For this review, take the finished solid that the model builds, in its own axes (mm). A direction names the side the tool comes from. Give positions to 0.01 mm unless a question says otherwise; leave off trailing zeros. Loops run counter-clockwise (first coordinate to the right, second up) from the corner with the lowest first, then second, coordinate; pieces in that order, holes last.
```python
from build123d import *

# Parameters (mm, degrees)
SKETCH2_W           = 45
SKETCH2_H           = 45
SKETCH2_R           = 11.5
SKETCH2_R_2         = 7.5
BOSS_EXTRUDE1_DEPTH = 4
SKETCH2_3_R         = 11.5
SKETCH2_3_R_2       = 7.5
BOSS_EXTRUDE2_DEPTH = 46
CHAMFER1_SIZE       = 10
SKETCH3_W           = 7
SKETCH3_H           = 20.450898806
CUT_EXTRUDE1_DEPTH  = 19


with BuildPart() as part:
    # Sketch2 → Boss-Extrude1 (new body)
    # profile 1 of 3: a face of its own
    with BuildSketch(Plane(origin=(0, 0, 0), x_dir=(1, 0, 0), z_dir=(0, 1, 0))):
        Rectangle(SKETCH2_W, SKETCH2_H)
        Circle(SKETCH2_R, mode=Mode.SUBTRACT)
    # profile 2 of 3: a face of its own
    with BuildSketch(Plane(origin=(0, 0, 0), x_dir=(1, 0, 0), z_dir=(0, 1, 0))):
        Circle(SKETCH2_R)
        Circle(SKETCH2_R_2, mode=Mode.SUBTRACT)
    # profile 3 of 3: a face of its own
    with BuildSketch(Plane(origin=(0, 0, 0), x_dir=(1, 0, 0), z_dir=(0, 1, 0))):
        Circle(SKETCH2_R_2)
    extrude(amount=-BOSS_EXTRUDE1_DEPTH)

    # Sketch2_3 → Boss-Extrude2 (add)
    with BuildSketch(Plane(origin=(0, 0, 0), x_dir=(1, 0, 0), z_dir=(0, 1, 0))):
        with Locations(Location((0, 0, 0), (0, 0, 270))):
            Circle(SKETCH2_3_R)
        with Locations(Location((0, 0, 0), (0, 0, 270))):
            Circle(SKETCH2_3_R_2, mode=Mode.SUBTRACT)
    extrude(amount=BOSS_EXTRUDE2_DEPTH)

    # Chamfer1
    chamfer1_edges = [part.edges().sort_by_distance(p)[0] for p in [
        (0, 0, -11.5),
    ]]
    chamfer(chamfer1_edges, length=CHAMFER1_SIZE)

    # Sketch3 → Cut-Extrude1 (cut)
    with BuildSketch(Plane.XY):
        with Locations((0, 21.362604589)):
            Rectangle(SKETCH3_W, SKETCH3_H)
    extrude(amount=CUT_EXTRUDE1_DEPTH, mode=Mode.SUBTRACT)


solid = part.part
```
Q1. Consider section A-A on x = 0. Give the boundary of the cut face in (y, z).
Answers:
outline: (-4, -22.5) - (0, -22.5) - (0, -21.5) - (10, -11.5) - (46, -11.5) - (46, -7.5) - (0, -7.5) - (0, 7.5) - (11.14, 7.5) - (11.14, 11.5) - (10, 11.5) - (0, 21.5) - (0, 22.5) - (-4, 22.5) - close; (31.59, 7.5) - (46, 7.5) - (46, 11.5) - (31.59, 11.5) - close
Q2. Consider section B-B on z = 0. Give the boundary of the cut face in (x, y).
Answers:
outline: (-22.5, -4) - (22.5, -4) - (22.5, 0) - (21.5, 0) - (11.5, 10) - (11.5, 46) - (7.5, 46) - (7.5, 0) - (-7.5, 0) - (-7.5, 46) - (-11.5, 46) - (-11.5, 10) - (-21.5, 0) - (-22.5, 0) - close
Q3. For probe 1 along X at (y, z) = (11, 0); probe 2 along Y at (x, z) = (19.5, 20); probe 3 along X at (y, z) = (17, 4), list the stretches that pass through material, from the lowest coordinate up.
Answers:
probe 1: x = -11.5 to -7.5, 7.5 to 11.5
probe 2: y = -4 to 0
probe 3: x = -10.78 to -6.34, 6.34 to 10.78
Q4. Mouldability with a two-part tool opening along Y and no side actions: class faces 4 (the flat face through (0, 11.137, 9)), 5 (the flat face through (0, 0, 0)), 6 (the flat face through (0, -4, 0)) as +Y half, -Y half, draft (parallel to the pull), parting line (faces both ways), or undercut.
Answers:
face 4: undercut
face 5: +Y half
face 6: -Y half
Q5. Consider section C-C on y = 34. Give the boundary of the cut face in (x, z), plus the area to 3 significant figures.
Answers:
outline: circle Ø23 at (0, 0); hole circle Ø15 at (0, 0)
area: 239 mm2
Q6. For pin 1 Ø1.3 at (y, z) = (22.5, 8.5) entering from +X; pin 2 Ø3 at (y, z) = (7, -6) entering from +X; pin 3 Ø17 at (x, z) = (0, 0) entering from +Y; pin 4 Ø2 at (y, z) = (25, 8.5) entering from -X, all flat-tipped, find the tip position at first contact; note any pin that passes through.
Answers:
pin 1: stops at x = 8.4
pin 2: stops at x = 14.93
pin 3: stops at y = 46
pin 4: stops at x = -8.72
Q7. Machinability: for faces 1 (the flat face through (22.5, -2, 0)), 2 (the flat face through (3.5, 21, 9)), 3 (the cylindrical face through (0.33, 22.678, -7.493)), which of the approach directions +Z, -Z, +X, -X, +Y, -Y give a long, thin tool a straight path to every point of the face, cutting with its end or side? Answer none if there is none.
Answers:
face 1: +Z, -Z, +X, +Y, -Y
face 2: +Z
face 3: +Y
